Read the model definition and answer for the solid it produces. Units are mm, in the model's axes. Coordinates: 2 decimals unless noted, no trailing zeros. Loops run counter-clockwise (first coordinate to the right, second up) from the corner with the lowest first, then second, coordinate; pieces in that order, holes last. Notation, with made-up numbers: (54.25, 5) -> (85.25, 5) arc R22 cw to (85.25, 40) -> close; hole circle Ø7 at (62, 43). An arc over 180 degrees is marked (long way). Answer in a Markdown table with one row per item.
```python
from build123d import *

# Parameters (mm, degrees)
BOSS_EXTRUDE1_DEPTH = 15
SKETCH4_R           = 2.54
CUT_EXTRUDE1_DEPTH  = 12.7
SKETCH5_R           = 2.54
CUT_EXTRUDE2_DEPTH  = 15.24
SKETCH6_W           = 50.620820664
SKETCH6_H           = 16.798394225
CUT_EXTRUDE3_DEPTH  = 15.24


with BuildPart() as part:
    # Sketch1 → Boss-Extrude1 (new body)
    with BuildSketch(Plane.XY):
        Polygon((-45.368681743, 5.31474447), (-45.781639963, 3.744360676), (-44.597190062, 2.280798517), (-42.364651707, 1.40510115), (-36.927606101, 0.59697268), (-26.918722281, 0), (-7.083221645, 0.593485987), (32.186093563, 4.677985502), (81.310277275, 12.243232279), (30.045684711, 13.095295678), (-9.952974473, 11.878999191), (-29.421950259, 9.844122216), (-38.797603286, 7.950869725), (-43.648710425, 6.454753464), align=None)
    extrude(amount=BOSS_EXTRUDE1_DEPTH)

    # Sketch4 → Cut-Extrude1 (cut)
    with BuildSketch(Plane(origin=(0, 0, 0), x_dir=(1, 0, 0), z_dir=(0, 1, 0))):
        with Locations(Location((-23.007190062, -7.5, 0), (0, 0, 180))):
            Circle(SKETCH4_R)
    extrude(amount=CUT_EXTRUDE1_DEPTH, mode=Mode.SUBTRACT)

    # Sketch5 → Cut-Extrude2 (cut)
    with BuildSketch(Plane(origin=(0, 0, 0), x_dir=(1, 0, 0), z_dir=(0, 1, 0))):
        with Locations(Location((12.552809938, -7.5, 0), (0, 0, 180))):
            Circle(SKETCH5_R)
    extrude(amount=CUT_EXTRUDE2_DEPTH, mode=Mode.SUBTRACT)

    # Sketch6 → Cut-Extrude3 (cut)
    with BuildSketch(Plane(origin=(0, 0, 0), x_dir=(1, 0, 0), z_dir=(0, 1, 0))):
        with Locations((57.506978049, -7.112855452)):
            Rectangle(SKETCH6_W, SKETCH6_H)
    extrude(amount=CUT_EXTRUDE3_DEPTH, mode=Mode.SUBTRACT)


solid = part.part
```
1. A cutting plane is placed at A-A on z = 6.5. Count the separate pieces of the cut face and the enclosed holes in it, and give its area (3 significant figures).
A:
| item | result |
|---|---|
| separate pieces | 3 |
| enclosed holes | 0 |
| area | 649 mm2 |
2. The mould has two halves that part along Z. Classify faces 1 (the flat face through (-31.993, 0.303, 7.395)), 2 (the cylindrical face through (10.206, 7.438, 6.527)), 3 (the flat face through (-7, 7, 0)), 4 (the cylindrical face through (-25.354, 5.348, 6.527)): pulls with the +Z half, pulls with the -Z half, needs draft (parallel to the pull), parting line crosses it, or undercut.
A:
| item | result |
|---|---|
| face 1 | needs draft |
| face 2 | undercut |
| face 3 | pulls with the -Z half |
| face 4 | undercut |
3. Given pin 1 Ø2 at (y, z) = (5.5, 7) entering from -X; pin 2 Ø5 at (x, z) = (-12.5, 4) entering from -Y, each flat-ended and moving along its own axis, determine where each tip first touches the part or whether it passes through.
A:
| item | result |
|---|---|
| pin 1 | stops at x = -45.58 |
| pin 2 | stops at y = 0.36 |
4. Find the intervals of material crossed by probe 1 along X at (y, z) = (6.25, 7.5); probe 2 along X at (y, z) = (5.75, 6); probe 3 along Z at (x, y) = (14.5, 3.25), in increasing order.
A:
| item | result |
|---|---|
| probe 1 | x = -43.96 to -25.55, -20.47 to 10.01, 15.09 to 32.2 |
| probe 2 | x = -44.71 to -25.06, -20.96 to 10.5, 14.6 to 32.2 |
| probe 3 | z = 0 to 5.87, 9.13 to 15 |
5. A cutting plane is placed at D-D on x = -11.5. Give the vertices of the cut face in (y, z), and give its area (3 significant figures).
A:
| item | result |
|---|---|
| outline | (0.46, 0) -> (11.72, 0) -> (11.72, 15) -> (0.46, 15) -> close |
| area | 169 mm2 |
6. A cutting plane is placed at C-C on x = -30.5. Give the vertices of the cut face in (y, z).
A:
| item | result |
|---|---|
| outline | (0.21, 0) -> (9.63, 0) -> (9.63, 15) -> (0.21, 15) -> close |
